from build123d import *

# Parameters (mm, degrees)
BOSS_EXTRUDE1_DEPTH          = 3.175
BOSS_EXTRUDE2_DEPTH          = 3.175
FILLET1_R                    = 1.27
BOSS_EXTRUDE3_DEPTH          = 41.275
FILLET1_OF_MIRROR2_R         = 1.27
BOSS_EXTRUDE4_DEPTH          = 12.7
F_18_0_1695_DIAMETER_HOLE1_D = 4.3053
CUT_EXTRUDE1_DEPTH           = 9.525
BOSS_EXTRUDE5_DEPTH          = 3.175
F_18_0_1695_DIAMETER_HOLE2_D = 4.3053


with BuildPart() as part:
    # Sketch1 → Boss-Extrude1 (new body)
    with BuildSketch(Plane(origin=(0, 0, 0), x_dir=(1, 0, 0), z_dir=(0, 1, 0))):
        Polygon((28.736819587, 28.736819587), (34.984785044, 28.736819587), (44.671604631, 19.05), (28.272599075, 19.05), (28.272599075, 0), (0, 0), align=None)
    boss_extrude1 = extrude(amount=BOSS_EXTRUDE1_DEPTH)

    # Mirror1: Boss-Extrude1 across plane
    add(boss_extrude1.mirror(Plane(origin=(0, 3.175, 0), x_dir=(-0.707106781, 0, 0.707106781), z_dir=(-0.707106781, 0, -0.707106781))))

    # Sketch2 → Boss-Extrude2 (add)
    with BuildSketch(Plane(origin=(0, 3.175, 0), x_dir=(1, 0, 0), z_dir=(0, 1, 0))):
        Polygon((29.11502011, 25.561819587), (29.11502011, 28.736819587), (34.984785044, 28.736819587), (44.671604631, 19.05), (40.181476571, 19.05), (33.669656983, 25.561819587), align=None)
    boss_extrude2 = extrude(amount=BOSS_EXTRUDE2_DEPTH)

    # Fillet1
    fillet1_edges = [part.edges().sort_by_distance(p)[0] for p in [
        (29.11502011, 4.7625, -28.736819587),
    ]]
    fillet(fillet1_edges, radius=FILLET1_R)

    # Sketch2_3 → Boss-Extrude3 (add)
    with BuildSketch(Plane(origin=(0, 3.175, 0), x_dir=(1, 0, 0), z_dir=(0, 1, 0))):
        Polygon((12.192, 0), (12.192, 12.192), (6.096, 6.096), align=None)
    boss_extrude3 = extrude(amount=BOSS_EXTRUDE3_DEPTH)

    # Mirror2: Boss-Extrude2, Boss-Extrude3 across plane
    add(boss_extrude2.mirror(Plane(origin=(0, 0, 0), x_dir=(-0.707106781, 0, 0.707106781), z_dir=(0.707106781, 0, 0.707106781))))
    add(boss_extrude3.mirror(Plane(origin=(0, 0, 0), x_dir=(-0.707106781, 0, 0.707106781), z_dir=(0.707106781, 0, 0.707106781))))

    # Fillet1 of Mirror2
    fillet1_of_mirror2_edges = [part.edges().sort_by_distance(p)[0] for p in [
        (28.736819587, 4.7625, -29.11502011),
    ]]
    fillet(fillet1_of_mirror2_edges, radius=FILLET1_OF_MIRROR2_R)

    # Sketch4 → Boss-Extrude4 (add)
    with BuildSketch(Plane(origin=(0, 44.45, 0), x_dir=(1, 0, 0), z_dir=(0, 1, 0))):
        Polygon((12.192, 0), (0, 12.192), (4.7625, 12.192), (12.192, 4.7625), align=None)
    extrude(amount=BOSS_EXTRUDE4_DEPTH)

    # 18 _0.1695_ Diameter Hole1 (through all)
    with Locations(Plane(origin=(8.47725, 0, -8.47725), x_dir=(-0.707106781, 0, -0.707106781), z_dir=(0.707106781, 0, -0.707106781))):
        with Locations((0, 52.3875)):
            Hole(F_18_0_1695_DIAMETER_HOLE1_D / 2)

    # Sketch7 → Cut-Extrude1 (cut)
    with BuildSketch(Plane(origin=(0, 3.175, 0), x_dir=(1, 0, 0), z_dir=(0, 1, 0))):
        Polygon((0, 0), (12.192, 0), (0, 12.192), align=None)
    extrude(amount=-CUT_EXTRUDE1_DEPTH, mode=Mode.SUBTRACT)

    # Sketch8 → Boss-Extrude5 (add)
    with BuildSketch(Plane(origin=(0, 0, 0), x_dir=(-1, 0, 0), z_dir=(0, -1, 0))):
        Polygon((-6.096, 6.096), (32.479604631, 44.671604631), (-19.05, 44.671604631), (-28.736819587, 34.984785044), (-28.736819587, 28.736819587), align=None)
    boss_extrude5 = extrude(amount=BOSS_EXTRUDE5_DEPTH)

    # Mirror3: Boss-Extrude5 across plane
    add(boss_extrude5.mirror(Plane(origin=(0, 0, 0), x_dir=(-0.707106781, 0, 0.707106781), z_dir=(0.707106781, 0, 0.707106781))))

    # 18 _0.1695_ Diameter Hole2 (through all)
    with Locations(Plane(origin=(0, -3.175, 0), x_dir=(-1, 0, 0), z_dir=(0, -1, 0))):
        with Locations((-34.924989631, -10.778219281)):
            f_18_0_1695_diameter_hole2 = Hole(F_18_0_1695_DIAMETER_HOLE2_D / 2)

    # Mirror4: 18 _0.1695_ Diameter Hole2 across plane
    add(f_18_0_1695_diameter_hole2.mirror(Plane(origin=(0, 0, 0), x_dir=(-0.707106781, 0, 0.707106781), z_dir=(0.707106781, 0, 0.707106781))), mode=Mode.SUBTRACT)


solid = part.part
Build history of the part. All positions in model axes, mm. A direction names the side the tool comes from. Coordinates: 2 decimals unless noted, no trailing zeros. Order: outer loops, then holes, each group sorted by start corner. A loop starts at its lowest first (then second) coordinate and runs counter-clockwise, first axis right, second up. Notation, with made-up numbers: (-10, 65.5) - (10, 65.5) arc R28 ccw to (10, 89.5) - close; hole circle Ø9 at (8.25, 36). An arc over 180 degrees is marked (long way). Put each result on its own line as item: value.
1. Drop flat-ended pins along their axis: P1, Ø1.9, axis at y = 2, z = -31, coming from the +X side; P2, Ø0.6, axis at y = 5.5, z = -26, coming from the -X side (3 decimals); P3, Ø3.5, axis at x = 21, y = 1, coming from the +Z side. Give the stop position or say it passes through.
Answer sheet:
P1: stops at x = 28.74
P2: stops at x = 29.115
P3: stops at z = 10.24
2. Probe line 1 along X through (y, z) = (3, -12.5); line 2 along Y through (x, z) = (14, -18) (3 decimals); line 3 along Y through (x, z) = (-7, -40) (3 decimals). List the from-to ranges inside material, lowest first. Write a range as [from, to].
Answer sheet:
line 1: x = [0, 28.27]
line 2: y = [-3.175, 3.175]
line 3: y = [-3.175, 0]
3. Saw through at A-A (y = 46.5). Write the cut outline in (x, z), and give its area (3 significant figures).
Answer sheet:
outline: (0, -12.19) - (4.76, -12.19) - (12.19, -4.76) - (12.19, 0) - close
area: 46.7 mm^2
4. Tool access for faces 1 (the face through (19.05, 2, -38)), 2 (the face through (12.192, 24, -6)), 3 (the face through (25.562, 5, -31)), 4 (the face through (0, 2, -20)): list every direction of +Z, -Z, +X, -X, +Y, -Y with a clear straight run to the whole face (end or side of a thin tool).
Answer sheet:
face 1: -Z, -X, +Y
face 2: +Z, -Z, +X, +Y
face 3: +Z, -X, +Y
face 4: +Z, -Z, -X, +Y
5. Pull direction Y, two halves, no side cores. Call faces 5 (the face through (8, 57.15, -8)), 6 (the face through (6.94, 50.286, -7.6)), 7 (the face through (-10.132, -1.565, -36.978)): pulls with the +Y half, pulls with the -Y half, needs draft (parallel to the pull), parting line crosses it, or undercut.
Answer sheet:
face 5: pulls with the +Y half
face 6: undercut
face 7: needs draft
6. Saw through at C-C (z = -2). Write the cut outline in (x, y) (3 decimals).
Answer sheet:
outline: (10.192, -3.175) - (44.672, -3.175) - (44.672, 0) - (28.273, 0) - (28.273, 3.175) - (12.192, 3.175) - (12.192, 57.15) - (10.192, 57.15) - close
7. Saw through at D-D (x = 2). Write the cut outline in (y, z) (3 decimals).
Answer sheet:
outline: (-3.175, -44.672) - (0, -44.672) - (0, -28.273) - (3.175, -28.273) - (3.175, -12.192) - (57.15, -12.192) - (57.15, -10.192) - (-3.175, -10.192) - close
